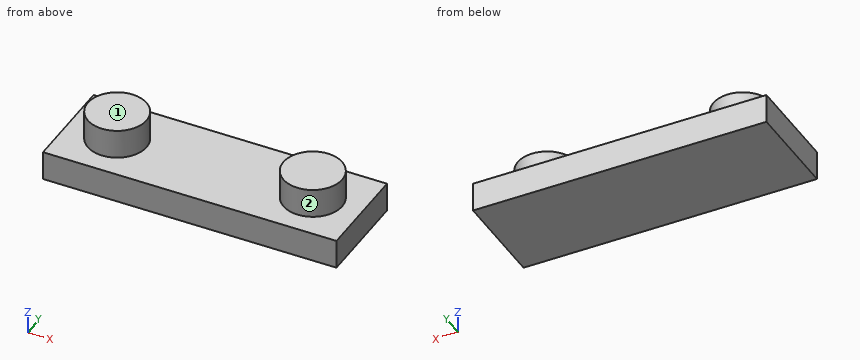
```python
from build123d import *

# Parameters (mm, degrees)
F0_W     = 30
F0_H     = 10
F0_R     = 3
F1_DEPTH = 3
F2_DEPTH = 6


with BuildPart() as f1:
    # F0 (on Top) → F1 (new body)
    with BuildSketch(Plane.XY):
        Rectangle(F0_W, F0_H)
        with Locations((-10, 0)):
            Circle(F0_R, mode=Mode.SUBTRACT)
        with Locations((10, 0)):
            Circle(F0_R, mode=Mode.SUBTRACT)
        with Locations((10, 0)):
            Circle(F0_R)
        with Locations((-10, 0)):
            Circle(F0_R)
    extrude(amount=F1_DEPTH)

    # F0 (on Top) → F2 (join)
    with BuildSketch(Plane.XY):
        with Locations((-10, 0)):
            Circle(F0_R)
        with Locations((10, 0)):
            Circle(F0_R)
    extrude(amount=F2_DEPTH)


solid = f1.part
```
Work out the finished part from the listing and answer in its coordinate system (mm). Face numbers are marked on the shaded views. A direction names the side the tool comes from. Round coordinates to 2 decimals unless told otherwise and drop trailing zeros. Loops run counter-clockwise (first coordinate to the right, second up) from the corner with the lowest first, then second, coordinate; pieces in that order, holes last. Notation, with made-up numbers: M 37.25,55 L 50.25,55 A26 ccw 50.25,74 Z; hole C 74,77 d6. An arc over 180 degrees is marked long. Use CSV: the item, a comma, the result in double quotes.
Q1. Section A-A, the plane y = 0 is taken. Determine the outline of the cut face in (x, z).
Determined:
outline,"M -15,0 L 15,0 L 15,3 L 13,3 L 13,6 L 7,6 L 7,3 L -7,3 L -7,6 L -13,6 L -13,3 L -15,3 Z"
Q2. A tool of negligible diameter and unlimited length cuts with its end or side. For the marked faces 1 and 2, from which of +Z, -Z, +X, -X, +Y, -Y can it reach the whole face along a straight path? Write none if from no direction.
Determined:
face 1,"+Z, +X, -X, +Y, -Y"
face 2,"+Z"
Q3. Section D-D, the plane x = -12.25 is taken. Determine the outline of the cut face in (y, z), then the cut area to 3 significant figures.
Determined:
outline,"M -5,0 L 5,0 L 5,3 L 1.98,3 L 1.98,6 L -1.98,6 L -1.98,3 L -5,3 Z"
area,"41.9 mm2"
Q4. Each of these flat-tipped pins is pushed along its axis until it touches: pin 1 (5 mm diameter, centred on x = 3, y = 1.5, fed in from +Z); pin 2 (5 mm diameter, centred on x = -10.5, y = 2, fed in from -Z). Where does it stop, or does it pass through?
Determined:
pin 1,"z = 3"
pin 2,"z = 0"
Q5. Section C-C, the plane x = 7.5 is taken. Determine the outline of the cut face in (y, z).
Determined:
outline,"M -5,0 L 5,0 L 5,3 L 1.66,3 L 1.66,6 L -1.66,6 L -1.66,3 L -5,3 Z"
Q6. Section B-B, the plane z = 4.2 is taken. Determine the outline of the cut face in (x, y).
Determined:
outline,"C -10,0 d6; C 10,0 d6"
Q7. Consider L1, parallel to Z at x = -8.5, y = -4; L2, parallel to X at y = -2.25, z = 5.4; L3, parallel to X at y = -0.5, z = 3.2. Determine where each line is inside the solid, lowest interval first.
Determined:
L1,"0 to 3"
L2,"-11.98 to -8.02, 8.02 to 11.98"
L3,"-12.96 to -7.04, 7.04 to 12.96"
